from build123d import *

# Parameters (mm, degrees)
SKETCH1_W           = 14
SKETCH1_H           = 12
BOSS_EXTRUDE1_DEPTH = 10
SKETCH2_R           = 5
BOSS_EXTRUDE2_DEPTH = 5
SKETCH3_R           = 5.25
BOSS_EXTRUDE3_DEPTH = 1
SKETCH5_R           = 4.5
CUT_EXTRUDE1_DEPTH  = 1.5
FILLET1_R           = 6
SKETCH11_R          = 1
BOSS_EXTRUDE4_DEPTH = 10


with BuildPart() as part:
    # Sketch1 → Boss-Extrude1 (new body)
    with BuildSketch(Plane(origin=(0, 0, 0), x_dir=(0, 0, -1), z_dir=(1, 0, 0))):
        Rectangle(SKETCH1_W, SKETCH1_H)
    extrude(amount=BOSS_EXTRUDE1_DEPTH)

    # Sketch2 → Boss-Extrude2 (add)
    with BuildSketch(Plane(origin=(10, 0, 0), x_dir=(0, 0, -1), z_dir=(1, 0, 0))):
        Circle(SKETCH2_R)
    extrude(amount=BOSS_EXTRUDE2_DEPTH)

    # Sketch3 → Boss-Extrude3 (add)
    with BuildSketch(Plane(origin=(15, 0, 0), x_dir=(0, 0, -1), z_dir=(1, 0, 0))):
        Circle(SKETCH3_R)
    extrude(amount=BOSS_EXTRUDE3_DEPTH)

    # Sketch5 → Cut-Extrude1 (cut)
    with BuildSketch(Plane(origin=(16, 0, 0), x_dir=(0, 0, -1), z_dir=(1, 0, 0))):
        Circle(SKETCH5_R)
    extrude(amount=-CUT_EXTRUDE1_DEPTH, mode=Mode.SUBTRACT)

    # Sketch6 → Revolve2 (revolve)
    with BuildSketch(Plane(origin=(0, 0, 0), x_dir=(1, 0, 0), z_dir=(0, 1, 0)), mode=Mode.PRIVATE) as revolve2_sk:
        with BuildLine():
            Line((11.6, 0), (15.6, 0))
            ThreePointArc((15.6, 0), (14.428427125, 2.828427125), (11.6, 4))
            Line((11.6, 4), (11.6, 0))
        make_face()
    revolve(revolve2_sk.sketch.rotate(Axis((11.6, 0, 0), (1, 0, 0)), 180), axis=Axis((11.6, 0, 0), (1, 0, 0)))

    # Fillet1
    fillet1_edges = [part.edges().sort_by_distance(p)[0] for p in [
        (0, -6, 0),
        (0, 6, 0),
    ]]
    fillet(fillet1_edges, radius=FILLET1_R - 0.0001)  # a hair under: the kernel refuses the full size

    # Sketch11 → Boss-Extrude4 (add, symmetric)
    with BuildSketch(Plane.XY):
        with Locations(Location((6, 0, 0), (0, 0, 90))):
            Circle(SKETCH11_R)
    extrude(amount=BOSS_EXTRUDE4_DEPTH, both=True)


solid = part.part
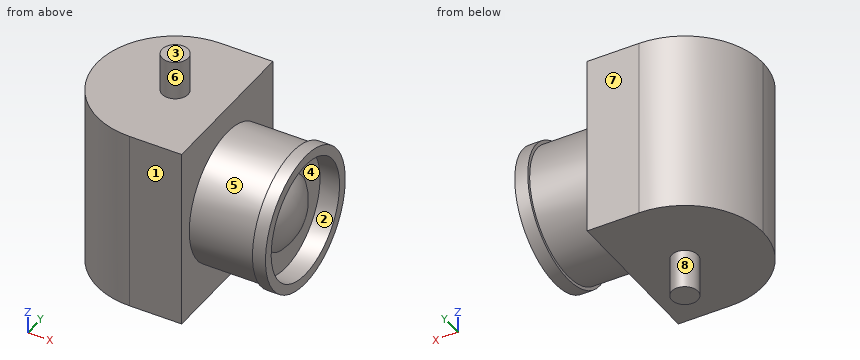
Geometry: final body of the model. Coordinates: model frame, mm. Face numbers are marked on the shaded views. A direction names the side the tool comes from. Coordinates: 2 decimals unless noted, no trailing zeros. Order: outer loops, then holes, each group sorted by start corner. A loop starts at its lowest first (then second) coordinate and runs counter-clockwise, first axis right, second up.
(1) First-contact query: pin 1 (1.5 mm diameter, centred on x = 2.5, y = 3, fed in from -Z); pin 2 (1 mm diameter, centred on x = 11.5, y = -3.5, fed in from +Z); pin 3 (3 mm diameter, centred on x = 4.5, y = 2.5, fed in from +Z). Flat tips, straight axial feed; report the tip coordinate or a pass-through.
(2) Material intervals for probe 1 along Z at (x, y) = (4.25, -5); probe 2 along Y at (x, z) = (15.2, 0); probe 3 along X at (y, z) = (0, -5.5), sorted ascending.
(3) Draft query along Z for the marked faces 1, 2, 3 and 4. Return one class per face: pulls with the +Z half, pulls with the -Z half, needs draft (parallel to the pull), parting line crosses it, or undercut.
(4) Access query for the marked faces 5, 6, 7 and 8. Directions: +Z, -Z, +X, -X, +Y, -Y. A direction counts if a zero-diameter tool reaches every point of the face in a straight line with its end or side. Return the directions, or none.
(5) Section query C-C (x = 8.5). Return the cut outline in (y, z), plus the area to 3 significant figures.
(6) Section query B-B (y = -3.25). Return the cut outline in (x, z), plus the area to 3 significant figures.
Solution:
1. pin 1: stops at z = -7
1. pin 2: stops at z = 4
1. pin 3: stops at z = 7
2. probe 1: z = -7 to 7
2. probe 2: y = -5.25 to -4.5, -1.74 to 1.74, 4.5 to 5.25
2. probe 3: x = 0 to 10
3. face 1: needs draft
3. face 2: undercut
3. face 3: pulls with the +Z half
3. face 4: undercut
4. face 5: none
4. face 6: +Z
4. face 7: +Z, -Z, +X, -X, +Y
4. face 8: -Z
5. outline: (-6, -7) - (6, -7) - (6, 7) - (-6, 7) - close
5. area: 168 mm2
6. outline: (0.96, -7) - (10, -7) - (10, -3.8) - (15, -3.8) - (15, -4.12) - (16, -4.12) - (16, -3.11) - (14.5, -3.11) - (14.5, 3.11) - (16, 3.11) - (16, 4.12) - (15, 4.12) - (15, 3.8) - (10, 3.8) - (10, 7) - (0.96, 7) - close
6. area: 164 mm2
